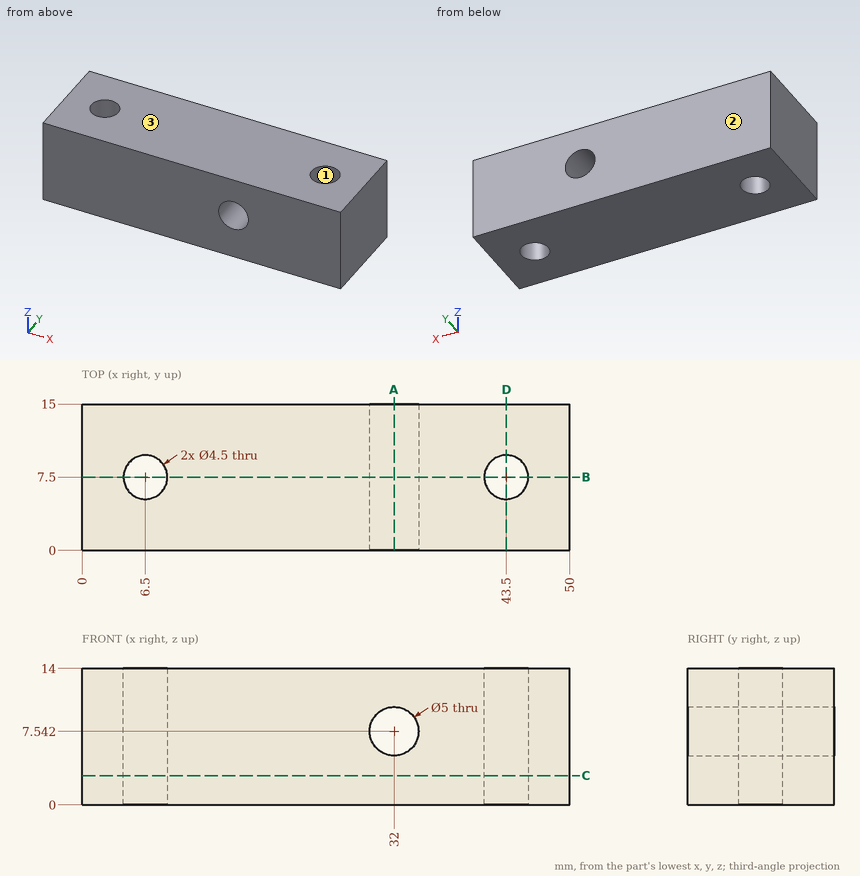
Part print with two shaded views. Sizes in mm from the minimum x, y, z corner. Coordinates: 2 decimals unless noted, no trailing zeros. Write each loop counter-clockwise with the first axis right and the second up, starting at its lowest first coordinate (ties: lowest second). Pieces come first, ordered by that corner, then holes. Notation, with made-up numbers: (34, 26.5) - (83, 26.5) arc R29 ccw to (83, 56.5) - close; hole circle Ø10 at (18.25, 53.5). An arc over 180 degrees is marked (long way). Use a Markdown table: item, result. Add a question column.
Item 1: Band-saw the part on D-D, the plane x = 43.5. Write the cut outline in (y, z).
Item 2: Drop a flat-ended pin along its axis: pin 1 (4 mm diameter, centred on x = 23.5, z = 6, fed in from -Y). Give the stop position or say it passes through.
Item 3: Band-saw the part on C-C, the plane z = 3. Write the cut outline in (x, y), and give its area (3 significant figures).
Item 4: Two-plate mould, pull along Y, no slides. Class the marked faces 1, 2 and 3: pulls with the +Y half, pulls with the -Y half, needs draft (parallel to the pull), parting line crosses it, or undercut.
Item 5: Drill centre lines: line 1 along Y through (x, z) = (43.5, 7.75); line 2 along Z through (x, y) = (32, 5); line 3 along X through (y, z) = (6.5, 11.25). Where is each one in solid material? Low to high.
Item 6: Band-saw the part on A-A, the plane x = 32. Write the cut outline in (y, z), and give its area (3 significant figures).
Item 7: Band-saw the part on B-B, the plane y = 7.5. Write the cut outline in (x, z), and give its area (3 significant figures).
A:
| question | item | result |
|---|---|---|
| 1 | outline | (0, 0) - (5.25, 0) - (5.25, 14) - (0, 14) - close; (9.75, 0) - (15, 0) - (15, 14) - (9.75, 14) - close |
| 2 | pin 1 | stops at y = 0 |
| 3 | outline | (0, 0) - (50, 0) - (50, 15) - (0, 15) - close; hole circle Ø4.5 at (6.5, 7.5); hole circle Ø4.5 at (43.5, 7.5) |
| 3 | area | 718 mm² |
| 4 | face 1 | undercut |
| 4 | face 2 | pulls with the +Y half |
| 4 | face 3 | needs draft |
| 5 | line 1 | y = 0 to 5.25, 9.75 to 15 |
| 5 | line 2 | z = 0 to 5.04, 10.04 to 14 |
| 5 | line 3 | x = 0 to 4.48, 8.52 to 41.48, 45.52 to 50 |
| 6 | outline | (0, 0) - (15, 0) - (15, 5.04) - (0, 5.04) - close; (0, 10.04) - (15, 10.04) - (15, 14) - (0, 14) - close |
| 6 | area | 135 mm² |
| 7 | outline | (0, 0) - (4.25, 0) - (4.25, 14) - (0, 14) - close; (8.75, 0) - (41.25, 0) - (41.25, 14) - (8.75, 14) - close; (45.75, 0) - (50, 0) - (50, 14) - (45.75, 14) - close; hole circle Ø5 at (32, 7.54) |
| 7 | area | 554 mm² |
